Could you check a few things on this model? Use its own coordinates, in mm. A direction names the side the tool comes from. Give positions to 0.01 mm unless a question says otherwise; leave off trailing zeros. Loops run counter-clockwise (first coordinate to the right, second up) from the corner with the lowest first, then second, coordinate; pieces in that order, holes last. Notation, with made-up numbers: (88, 30.5) -> (99, 30.5) arc R24 ccw to (99, 67.5) -> close; hole circle Ø3 at (2, 25). An arc over 180 degrees is marked (long way). Put each result on its own line as item: value.
```python
from build123d import *

# Parameters (mm, degrees)
BOSS_EXTRUDE1_DEPTH = 22.5
SKETCH2_R           = 2.5
CUT_EXTRUDE1_DEPTH  = 51.759851261
CHAMFER1_SIZE       = 1.75
FILLET1_R           = 1
CHAMFER2_SIZE       = 1


with BuildPart() as part:
    # Sketch1 → Boss-Extrude1 (new, symmetric)
    with BuildSketch(Plane.XY):
        Polygon((0, -10.625), (0, 10.625), (4.5, 10.625), (4.5, 7.125), (13.25, 7.125), (13.25, 13.75), (36.25, 13.75), (36.25, 9.75), (19.25, 9.75), (19.25, -9.75), (36.25, -9.75), (36.25, -13.75), (13.25, -13.75), (13.25, -7.125), (4.5, -7.125), (4.5, -10.625), align=None)
    extrude(amount=BOSS_EXTRUDE1_DEPTH, both=True)

    # Sketch2 → Cut-Extrude1 (cut, through all)
    with BuildSketch(Plane.XZ.offset(13.75)):
        with Locations(Location((30.25, 15.5, 0), (0, 0, 270))):
            Circle(SKETCH2_R)
        with Locations(Location((24.25, 0, 0), (0, 0, 270))):
            Circle(SKETCH2_R)
        with Locations(Location((30.25, -15.5, 0), (0, 0, 270))):
            Circle(SKETCH2_R)
    extrude(amount=-CUT_EXTRUDE1_DEPTH, mode=Mode.SUBTRACT)

    # Chamfer1
    chamfer1_edges = [part.edges().sort_by_distance(p)[0] for p in [
        (30.25, 13.75, 18),
        (30.25, -13.75, 18),
        (24.25, 13.75, 2.5),
        (24.25, -13.75, 2.5),
        (30.25, 13.75, -13),
        (30.25, -13.75, -13),
    ]]
    chamfer(chamfer1_edges, length=CHAMFER1_SIZE)

    # Fillet1
    fillet1_edges = [part.edges().sort_by_distance(p)[0] for p in [
        (4.5, 10.625, 0),
        (4.5, 7.125, 0),
        (13.25, 7.125, 0),
        (13.25, 13.75, 0),
        (36.25, 13.75, 0),
        (36.25, 9.75, 0),
        (19.25, 9.75, 0),
        (19.25, -9.75, 0),
        (36.25, -9.75, 0),
        (36.25, -13.75, 0),
        (13.25, -13.75, 0),
        (13.25, -7.125, 0),
        (4.5, -7.125, 0),
        (4.5, -10.625, 0),
        (0, -10.625, 0),
        (0, 10.625, 0),
    ]]
    fillet(fillet1_edges, radius=FILLET1_R)

    # Chamfer2
    chamfer2_edges = [part.edges().sort_by_distance(p)[0] for p in [
        (0, 0, -22.5),
        (4.207106781, -10.332106781, -22.5),
        (0.292893219, 10.332106781, -22.5),
        (0.292893219, -10.332106781, -22.5),
        (13.542893219, -13.457106781, -22.5),
        (35.957106781, -13.457106781, -22.5),
        (35.957106781, -10.042893219, -22.5),
        (35.957106781, 10.042893219, -22.5),
        (35.957106781, 13.457106781, -22.5),
        (13.542893219, 13.457106781, -22.5),
        (4.207106781, 10.332106781, -22.5),
        (4.5, 8.875, 22.5),
        (0, 0, 22.5),
        (2.25, -10.625, 22.5),
        (4.5, -8.875, 22.5),
        (8.875, -7.125, 22.5),
        (13.25, -10.4375, 22.5),
        (24.75, -13.75, 22.5),
        (36.25, -11.75, 22.5),
        (27.75, -9.75, 22.5),
        (19.25, 0, 22.5),
        (27.75, 9.75, 22.5),
        (36.25, 11.75, 22.5),
        (24.75, 13.75, 22.5),
        (13.25, 10.4375, 22.5),
        (8.875, 7.125, 22.5),
        (4.207106781, -10.332106781, 22.5),
        (0.292893219, 10.332106781, 22.5),
        (0.292893219, -10.332106781, 22.5),
        (13.542893219, -13.457106781, 22.5),
        (35.957106781, -13.457106781, 22.5),
        (35.957106781, -10.042893219, 22.5),
        (35.957106781, 10.042893219, 22.5),
        (35.957106781, 13.457106781, 22.5),
        (13.542893219, 13.457106781, 22.5),
        (4.207106781, 10.332106781, 22.5),
        (4.792893219, 7.417893219, -22.5),
        (4.792893219, 7.417893219, 22.5),
        (12.957106781, 7.417893219, -22.5),
        (12.957106781, 7.417893219, 22.5),
        (19.542893219, 9.457106781, -22.5),
        (19.542893219, 9.457106781, 22.5),
        (19.542893219, -9.457106781, -22.5),
        (19.542893219, -9.457106781, 22.5),
        (12.957106781, -7.417893219, -22.5),
        (12.957106781, -7.417893219, 22.5),
        (4.792893219, -7.417893219, -22.5),
        (4.792893219, -7.417893219, 22.5),
        (2.25, 10.625, -22.5),
        (2.25, 10.625, 22.5),
        (4.5, 8.875, -22.5),
        (8.875, 7.125, -22.5),
        (13.25, 10.4375, -22.5),
        (24.75, 13.75, -22.5),
        (36.25, 11.75, -22.5),
        (27.75, 9.75, -22.5),
        (19.25, 0, -22.5),
        (27.75, -9.75, -22.5),
        (36.25, -11.75, -22.5),
        (24.75, -13.75, -22.5),
        (13.25, -10.4375, -22.5),
        (8.875, -7.125, -22.5),
        (4.5, -8.875, -22.5),
        (2.25, -10.625, -22.5),
    ]]
    chamfer(chamfer2_edges, length=CHAMFER2_SIZE)


solid = part.part
```
1. I need wall thicknesses on line 1 (X direction, y = -10.8, z = 15.5); line 2 (Y direction, x = 23, z = 18). Which ranges of each line are inside material? Lowest first, please.
Recorded:
line 1: x = 13.25 to 27.75, 32.75 to 36.25
line 2: y = -13.75 to -9.75, 9.75 to 13.75
2. I'm going to push flat-ended pins straight in: pin 1 (6.5 mm diameter, centred on x = 24.25, z = 0, fed in from -Y); pin 2 (12 mm diameter, centred on x = 31.5, y = 7.5, fed in from -Z); pin 3 (1.4 mm diameter, centred on y = -11.5, z = 8.5, fed in from -X); pin 4 (4 mm diameter, centred on x = 30.25, z = -15.5, fed in from +Y). Where does each tip first touch, or does it pass through?
Recorded:
pin 1: stops at y = -12.75
pin 2: stops at z = -22.5
pin 3: stops at x = 13.25
pin 4: passes through
3. For faces 1 (the face through (27.64, -10.24, -21.99)), 2 (the face through (9, -7.125, 0)), 3 (the face through (4.51, 7.16, 21.88)), which set-ups out of +Z, -Z, +X, -X, +Y, -Y let a thin tool reach every point of the face, with its end or its side?
Recorded:
face 1: -Z, +X
face 2: +Z, -Z, -Y
face 3: +Z, +Y
4. Thinking about a two-plate mould opening in Y: for faces 4 (the face through (18.76, 0.12, 21.99)), 5 (the face through (31.94, 10.86, -13.66)), 6 (the face through (35.605, 13.112, -21.993)), which applies, pulls with the +Y half, pulls with the -Y half, needs draft (parallel to the pull), parting line crosses it, or undercut?
Recorded:
face 4: undercut
face 5: needs draft
face 6: pulls with the +Y half
5. If we section it at C-C (z = -15.5): Count the separate pieces of the cut face and the enclosed holes in it, then the cut area to 3 significant figures.
Recorded:
separate pieces: 3
enclosed holes: 0
area: 474 mm^2
6. If we section it at A-A (x = 24.25): List the corners of the cut face in (y, z) for me.
Recorded:
outline: (-13.75, -21.5) -> (-12.75, -22.5) -> (-10.75, -22.5) -> (-9.75, -21.5) -> (-9.75, -2.5) -> (-12, -2.5) -> (-13.75, -4.25) -> close; (-13.75, 4.25) -> (-12, 2.5) -> (-9.75, 2.5) -> (-9.75, 21.5) -> (-10.75, 22.5) -> (-12.75, 22.5) -> (-13.75, 21.5) -> close; (9.75, -21.5) -> (10.75, -22.5) -> (12.75, -22.5) -> (13.75, -21.5) -> (13.75, -4.25) -> (12, -2.5) -> (9.75, -2.5) -> close; (9.75, 2.5) -> (12, 2.5) -> (13.75, 4.25) -> (13.75, 21.5) -> (12.75, 22.5) -> (10.75, 22.5) -> (9.75, 21.5) -> close
7. If we section it at B-B (y = -4.5): List the corners of the cut face in (x, z) for me, then the cut area to 3 significant figures.
Recorded:
outline: (0, -21.5) -> (1, -22.5) -> (18.25, -22.5) -> (19.25, -21.5) -> (19.25, 21.5) -> (18.25, 22.5) -> (1, 22.5) -> (0, 21.5) -> close
area: 864 mm^2
